Check sheet for the modelled part. Datum: model origin and axes. Units: mm. Round coordinates to 2 decimals unless told otherwise and drop trailing zeros. Order: outer loops, then holes, each group sorted by start corner. A loop starts at its lowest first (then second) coordinate and runs counter-clockwise, first axis right, second up.
Q1. Depth check by flat-ended pin: P1, Ø6, axis at y = 26, z = 17, coming from the +X side; P2, Ø2, axis at x = -53, z = 39.5, coming from the +Y side; P3, Ø5, axis at x = -33.5, y = 14.5, coming from the -Z side; P4, Ø8, axis at x = 46, z = 24.5, coming from the +Y side. Enter the tip coordinate at first touch or a pass-through.
Q2. Cross-section at B-B on x = 0. Record the cut outline in (y, z), then the cut area to 3 significant figures.
Q3. Cross-section at C-C on z = 56. Record the cut outline in (x, y).
Q4. Cross-section at D-D on z = 70. Record the cut outline in (x, y), then the cut area to 3 significant figures.
Q5. Cross-section at A-A on z = 29. Record the cut outline in (x, y), then the cut area to 3 significant figures.
Q6. Mould release check, pull along X, two halves, no side actions. Record for faces 1 (the conical face through (0.498, 22.646, 37.03)), 2 (the conical face through (0.7, 31.82, 62.95)), 3 (the flat face through (1, 24, 0)), 4 (the conical face through (1.457, 66.244, 37.906)): +X half, -X half, draft (parallel to the pull), parting line (faces both ways), or undercut.
Q7. Scan lines: probe 1 along X at (y, z) = (3, 37.5); probe 2 along Y at (x, z) = (-9, 36.5) (1 decimal); probe 3 along Z at (x, y) = (-25.5, 39). Record each from-to range of solid material in increasing order.
from build123d import *

# Parameters (mm, degrees)
F1_ANGLE = 180


# Not quite as in the source:
# - the program builds the solid bodies; features that only make, move or delete a surface that nothing else refers to are left out


with BuildPart() as f1:
    # F0 (on Front) → F1 (revolve)
    with BuildSketch(Plane.XZ):
        Polygon((12.4851092696, 39.2489619553), (0, 15.0755345821), (0, 0), (61.1490756273, 0), (71.2305568159, 74.7646316886), (29.8195946962, 62.3483546078), (15.6820116428, 12.4102499136), align=None)
    revolve(axis=Axis((0, 0, 7.5377672911), (0, 0, 1)), revolution_arc=F1_ANGLE)


solid = f1.part
Results found:
1. P1: stops at x = 59.2
1. P2: stops at y = 41.43
1. P3: stops at z = 0
1. P4: stops at y = 48.96
2. outline: (0, 0) - (61.15, 0) - (71.23, 74.76) - (29.82, 62.35) - (15.68, 12.41) - (12.49, 39.25) - (0, 15.08) - close
2. area: 3,410 mm2
3. outline: (-68.7, 0) - (-28.02, 0) arc R28.02 cw to (28.02, 0) - (68.7, 0) arc R68.7 ccw to start
4. outline: (-70.59, 0) - (-55.34, 0) arc R55.34 cw to (55.34, 0) - (70.59, 0) arc R70.59 ccw to start
4. area: 3,020 mm2
5. outline: (-65.06, 0) - (-20.38, 0) arc R20.38 cw to (20.38, 0) - (65.06, 0) arc R65.06 ccw to start; (-13.71, 0) - (-7.19, 0) arc R7.19 cw to (7.19, 0) - (13.71, 0) arc R13.71 ccw to start
5. area: 6,210 mm2
6. face 1: undercut
6. face 2: undercut
6. face 3: draft
6. face 4: parting line
7. probe 1: x = -66.14 to -22.59, -12.33 to -11.19, 11.19 to 12.33, 22.59 to 66.14
7. probe 2: y = 6.4 to 9.1, 20.6 to 65.5
7. probe 3: z = 0 to 67.38
